Verification items for the finished model (mm, model axes). Face numbers are marked on the shaded views. A direction names the side the tool comes from. Coordinates: 2 decimals unless noted, no trailing zeros. Loops run counter-clockwise (first coordinate to the right, second up) from the corner with the lowest first, then second, coordinate; pieces in that order, holes last. Notation, with made-up numbers: (-25.75, 8) - (7.25, 8) arc R20 ccw to (7.25, 18) - close; hole circle Ø1 at (83.5, 3). An arc over 180 degrees is marked (long way). One line per item, written item: value. Start each with the question number.
(1) Thickness scan on probe 1 along Z at (x, y) = (10, 19); probe 2 along Y at (x, z) = (0, 1.6); probe 3 along X at (y, z) = (-20, 13.5). Record the ranges inside material, lowest first. Write a range as [from, to].
(2) Section check D-D (x = 43). Record the boundary of the cut face in (y, z), plus the area to 3 significant figures.
(3) Set-up check for the marked faces 1, 2 and 3: record each of +Z, -Z, +X, -X, +Y, -Y from which the full face is reachable in a straight line by a thin tool's end or side.
(4) Gauge pin test, flat ends, axial feed: P1, Ø4, axis at y = 43.5, z = 2.5, coming from the -X side; P2, Ø3.5, axis at y = -30, z = 64, coming from the -X side; P3, Ø2.5, axis at x = -46.5, z = 2.5, coming from the -Y side; P4, Ø8, axis at x = 37.5, y = 21.5, coming from the -Z side. Record the tip position at first contact, or that the pin passes through.
(5) Section check A-A (z = 43.5). Record the boundary of the cut face in (x, y), plus the area to 3 significant figures.
(6) Draft check along Z on the marked faces 4, 5 and 6. Enter one of: +Z half, -Z half, draft (parallel to the pull), parting line (faces both ways), or undercut.
(7) Section check C-C (x = 0). Record the boundary of the cut face in (y, z), plus the area to 3 significant figures.
(8) Section check B-B (y = 0). Record the boundary of the cut face in (x, z).
Autodesk Inventor part; units mm, degrees
ref_plane "YZ Plane" through (0, 0, 0) normal (1, 0, 0) x (0, 1, 0)
ref_plane "XZ Plane" through (0, 0, 0) normal (0, 1, 0) x (-1, 0, 0)
ref_plane "XY Plane" through (0, 0, 0) normal (0, 0, 1) x (1, 0, 0)
sketch "Sketch1" plane through (0, 0, 0) normal (0, 0, 1) x (1, 0, 0)
  circle A0 centre (0, 0) radius 40.5
  line L0 (0, 0) -> (0, 50) construction
  arc A1 (6, 50) -> (-6, 50) centre (0, 50) ccw
  line L1 (0, 0) -> (50, 0) construction
  arc A2 (50, -6) -> (50, 6) centre (50, 0) ccw
  line L2 (0, 0) -> (-50, 0) construction
  arc A3 (-50, 6) -> (-50, -6) centre (-50, 0) ccw
  line L3 (-6, 50) -> (-6, 40.0531)
  line L4 (6, 40.0531) -> (6, 50)
  line L5 (-40.0531, 6) -> (-50, 6)
  line L6 (-50, -6) -> (-40.0531, -6)
  line L7 (50, 6) -> (40.0531, 6)
  line L8 (40.0531, -6) -> (50, -6)
  circle A4 centre (-50, 0) radius 1.75
  circle A5 centre (0, 50) radius 1.75
  circle A6 centre (50, 0) radius 1.75
  point P0 (0, 25)
  point P1 (25, 0)
  point P2 (-25, 0)
  dimension "d0" = 81
  dimension "d3" = 50
  dimension "d4" = 12
  dimension "d5" = 50
  dimension "d6" = 12
  dimension "d7" = 50
  dimension "d8" = 12
  dimension "d9" = 3.5
  dimension "d10" = 3.5
  dimension "d11" = 3.5
extrude "Extrusion2" add sketch "Sketch1" along normal blind 5
sketch "Sketch2" plane through (0, 0, 5) normal (0, 0, 1) x (1, 0, 0)
  arc A0 (-40.0531, -6) -> (40.0531, -6) centre (0, 0) ccw
  line L0 (-40.0531, -6) -> (-40.0531, -6)
  line L1 (-40.0531, -6) -> (-40.0531, -6) construction
  line L2 (-30.0531, -16) -> (-30.0531, -17.1489)
  line L3 (40.0531, -6) -> (40.0531, -6)
  line L4 (30.0531, -16) -> (30.0531, -17.1489)
  arc A1 (-30.0531, -17.1489) -> (-20.0531, -27.1489) centre (-20.0531, -17.1489) ccw
  arc A2 (20.0531, -27.1489) -> (30.0531, -17.1489) centre (20.0531, -17.1489) ccw
  arc A3 (40.0531, -6) -> (30.0531, -16) centre (40.0531, -16) ccw
  arc A4 (-30.0531, -16) -> (-40.0531, -6) centre (-40.0531, -16) ccw
  line L5 (-3, -27.1489) -> (-3, -40.3887)
  line L6 (3, -27.1489) -> (3, -40.3887)
  line L7 (20.0531, -27.1489) -> (3, -27.1489)
  line L8 (-3, -27.1489) -> (-20.0531, -27.1489)
  point P0 (-30.0531, -6)
  point P1 (-30.0531, -27.1489)
  point P2 (30.0531, -6)
  point P3 (30.0531, -27.1489)
  dimension "d16" = 10
  dimension "d17" = 0
  dimension "d18" = 90
  dimension "d19" = 10
  dimension "d20" = 10
extrude "Extrusion3" add sketch "Sketch2" along normal blind 60
sketch "Sketch3" plane through (0, 0, 65) normal (0, 0, 1) x (1, 0, 0)
  arc A0 (3, -40.3621) -> (-3, -40.3621) centre (0, 0) ccw
  arc A1 (6, 50) -> (-6, 50) centre (0, 50) ccw
  line L0 (0, 0) -> (0, 50) construction
  line L1 (6, 0) -> (6, 50)
  line L2 (-6, 50) -> (-6, 0)
  arc A2 (-6, 0) -> (6, 0) centre (0, 0) ccw
  arc A3 (6, 50) -> (-6, 50) centre (0, 50) ccw
  line L3 (0, 0) -> (50, 0) construction
  line L4 (0, 0) -> (50, 0) construction
  line L5 (0, -6) -> (50, -6)
  line L6 (50, 6) -> (0, 6)
  arc A4 (0, 6) -> (0, -6) centre (0, 0) ccw
  arc A5 (50, -6) -> (50, 6) centre (50, 0) ccw
  line L7 (0, 0) -> (-50, 0) construction
  line L8 (0, 6) -> (-50, 6)
  line L9 (-50, -6) -> (0, -6)
  arc A6 (0, -6) -> (0, 6) centre (0, 0) ccw
  arc A7 (-50, 6) -> (-50, -6) centre (-50, 0) ccw
  circle A8 centre (50, 0) radius 1.75
  circle A9 centre (-50, 0) radius 1.75
  circle A10 centre (0, 50) radius 1.75
  line L10 (-3, -40.3887) -> (-3, -36.6883)
  line L11 (3, -36.6883) -> (3, -40.3887)
  arc A11 (3, -36.6883) -> (-3, -36.6883) centre (0, -27.1489) ccw
  point P0 (0, 25)
  point P1 (25, 0)
  point P2 (-25, 0)
  dimension "d26" = 50
  dimension "d27" = 90
  dimension "d28" = 12
  dimension "d29" = 50
  dimension "d30" = 12
  dimension "d31" = 50
  dimension "d32" = 12
  dimension "d33" = 3.5
  dimension "d34" = 3.5
  dimension "d35" = 3.5
  dimension "d45" = 20
extrude "Extrusion4" add sketch "Sketch3" along normal blind 5
sketch "Sketch4" plane through (3, -27.1489, 5) normal (0, 1, 0) x (1, 0, 0)
  line L0 (7, -60) -> (0, -60)
  line L1 (-6, -60) -> (-13, -60)
  line L2 (0, -70) -> (5, -70)
  line L3 (5, -70) -> (13, -70) construction
  line L4 (-6, -60) -> (-43.0263, -60)
  line L5 (-11, -70) -> (-3, -70) construction
  line L6 (7, -60) -> (-13, -60)
  line L7 (-13, -60) -> (-13, -52)
  line L8 (-13, -52) -> (7, -52)
  line L9 (7, -52) -> (7, -60)
  line L10 (7, -60) -> (-13, -60)
  line L11 (-13, -60) -> (-13, -65)
  line L12 (-13, -65) -> (7, -65)
  line L13 (7, -65) -> (7, -60)
  point P0 (-3, 5)
  point P1 (0, -60)
  dimension "d46" = 8
  dimension "d47" = 20
  dimension "d48" = 5
extrude "Extrusion5" cut sketch "Sketch4" against normal blind 15
ref_plane "Work Plane1" through (0, 0, 65) normal (-1, 0, 0) x (0, 1, 0)
properties part number "Astra_slot"
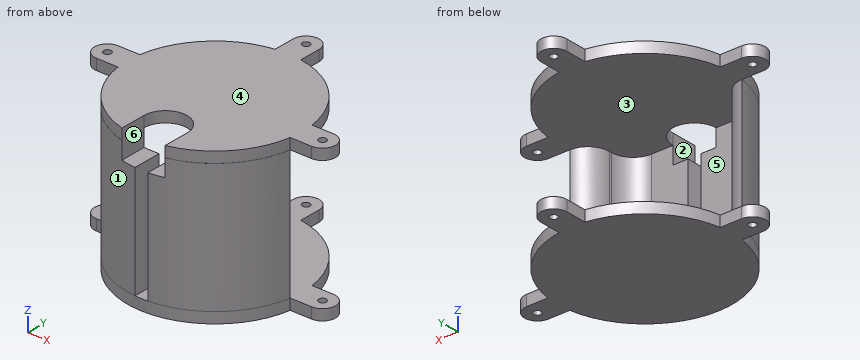
Responses:
1. probe 1: z = [0, 5], [65, 70]
1. probe 2: y = [-40.5, 48.25], [51.75, 56]
1. probe 3: x = [-35.22, -29.64], [29.64, 35.22]
2. outline: (-6, 0) - (6, 0) - (6, 5) - (-6, 5) - close; (-6, 65) - (6, 65) - (6, 70) - (-6, 70) - close
2. area: 120 mm²
3. face 1: +Z, -Z, -X, -Y
3. face 2: +Z, -Y
3. face 3: +Y
4. P1: stops at x = -6
4. P2: stops at x = -29.02
4. P3: stops at y = -6
4. P4: stops at z = 0
5. outline: (-40.05, -6) arc R40.5 ccw to (-3, -40.39) - (-3, -27.15) - (-20.05, -27.15) arc R10 cw to (-30.05, -17.15) - (-30.05, -16) arc R10 ccw to start; (3, -40.39) arc R40.5 ccw to (40.05, -6) arc R10 ccw to (30.05, -16) - (30.05, -17.15) arc R10 cw to (20.05, -27.15) - (3, -27.15) - close
5. area: 741 mm²
6. face 4: +Z half
6. face 5: undercut
6. face 6: draft
7. outline: (-40.5, 0) - (48.25, 0) - (48.25, 5) - (-40.5, 5) - close; (-17.15, 65) - (48.25, 65) - (48.25, 70) - (-17.15, 70) - close; (51.75, 0) - (56, 0) - (56, 5) - (51.75, 5) - close; (51.75, 65) - (56, 65) - (56, 70) - (51.75, 70) - close
7. area: 813 mm²
8. outline: (-56, 0) - (-51.75, 0) - (-51.75, 5) - (-56, 5) - close; (-56, 65) - (-51.75, 65) - (-51.75, 70) - (-56, 70) - close; (-48.25, 0) - (48.25, 0) - (48.25, 5) - (-48.25, 5) - close; (-48.25, 65) - (48.25, 65) - (48.25, 70) - (-48.25, 70) - close; (51.75, 0) - (56, 0) - (56, 5) - (51.75, 5) - close; (51.75, 65) - (56, 65) - (56, 70) - (51.75, 70) - close
